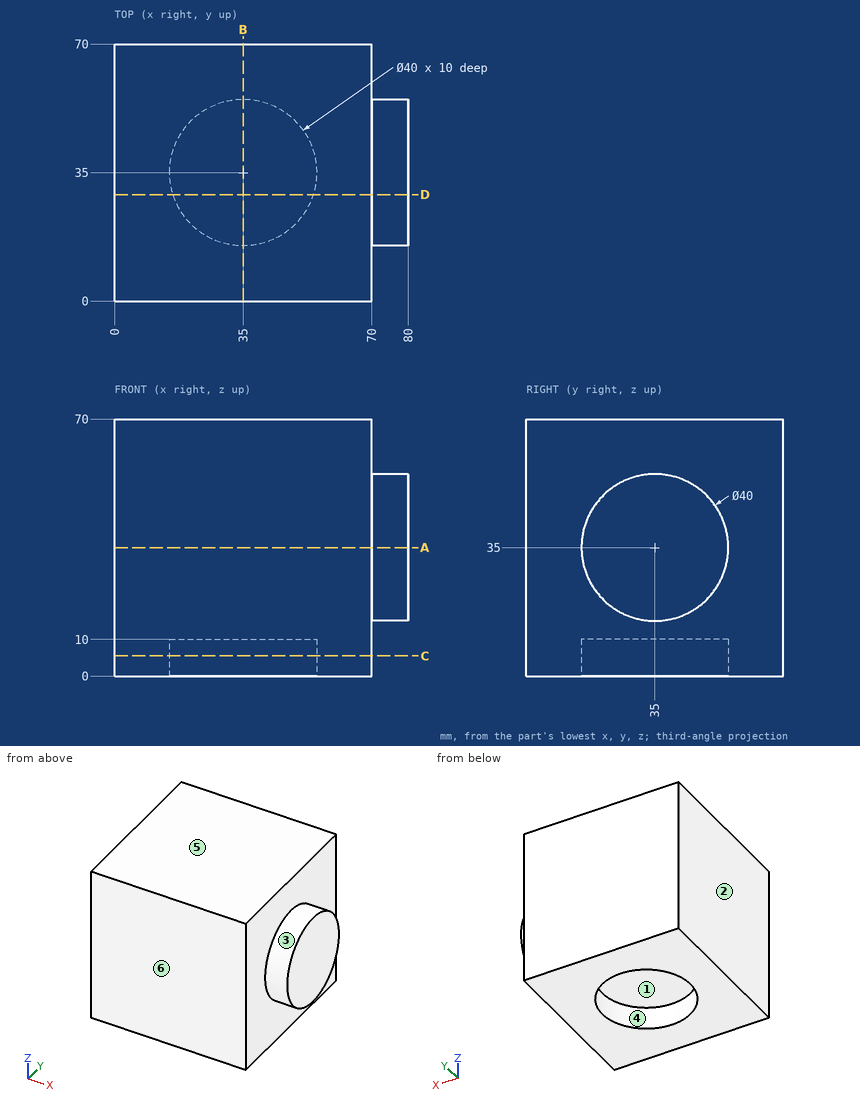
Design review of the part shown in the three views and the two pictorial views. Dimensions are in mm from the part's minimum x, y and z. A direction names the side the tool comes from. Give positions to 0.01 mm unless a question says otherwise; leave off trailing zeros. Write each loop counter-clockwise with the first axis right and the second up, starting at its lowest first coordinate (ties: lowest second). Pieces come first, ordered by that corner, then holes. Notation, with made-up numbers: M 47,0.5 L 95,0.5 A26 ccw 95,39.5 Z; hole C 39,4.5 d5. An arc over 180 degrees is marked long. One line per item, written item: value.
1) Take a section at A-A, the plane z = 35. Write out the cut boundary in (x, y).
Results are:
outline: M 0,0 L 70,0 L 70,15 L 80,15 L 80,55 L 70,55 L 70,70 L 0,70 Z
2) The part is to be moulded in two halves that separate along Y. For the marked faces 4, 5 and 6, say which applies: +Y half, -Y half, draft (parallel to the pull), parting line (faces both ways), or undercut.
Results are:
face 4: undercut
face 5: draft
face 6: -Y half
3) Take a section at C-C, the plane z = 5.5. Write out the cut boundary in (x, y).
Results are:
outline: M 0,0 L 70,0 L 70,70 L 0,70 Z; hole C 35,35 d40
4) For the marked faces 1, 2 and 3, list the 3-axis set-ups (+Z, -Z, +X, -X, +Y, -Y) from which the entire face can be reached by the end or side of a thin tool; tool diameter is ignored.
Results are:
face 1: -Z
face 2: +Z, -Z, -X, +Y, -Y
face 3: +X
5) Take a section at B-B, the plane x = 35. Write out the cut boundary in (y, z), then the cut area to 3 significant figures.
Results are:
outline: M 0,0 L 15,0 L 15,10 L 55,10 L 55,0 L 70,0 L 70,70 L 0,70 Z
area: 4,500 mm²
6) For line 1 (Y direction, x = 35, z = 7); line 2 (X direction, y = 31, z = 14); line 3 (Z direction, x = 35, y = 18), list the stretches that pass through material, from the lowest coordinate up. Write a range as from..to.
Results are:
line 1: y = 0..15, 55..70
line 2: x = 0..70
line 3: z = 10..70
7) For P1, Ø20, axis at x = 34.5, y = 32.5, coming from the -Z side; P2, Ø1.5, axis at x = 72, y = 19, coming from the +Z side, all flat-tipped, find the tip position at first contact; note any pin that passes through.
Results are:
P1: stops at z = 10
P2: stops at z = 47.94
8) Take a section at D-D, the plane y = 29. Write out the cut boundary in (x, z).
Results are:
outline: M 0,0 L 15.92,0 L 15.92,10 L 54.08,10 L 54.08,0 L 70,0 L 70,15.92 L 80,15.92 L 80,54.08 L 70,54.08 L 70,70 L 0,70 Z
